Work out the finished part from the listing and answer in its coordinate system (mm). A direction names the side the tool comes from. Round coordinates to 2 decimals unless told otherwise and drop trailing zeros. Write each loop counter-clockwise with the first axis right and the second up, starting at its lowest first coordinate (ties: lowest second). Pieces come first, ordered by that corner, then holes. Notation, with made-up numbers: M 54.5,66.5 L 80.5,66.5 A32 cw 80.5,92.5 Z; hole C -39.75,18.5 d11. An arc over 180 degrees is marked long. One line per item, written item: value. Start each with the question number.
Q1. Find section A-A (y = -85). Write down the section's boundary in (x, z).
Q2. Find section B-B (x = -120.5). Write down the section's boundary in (y, z), and give its area (3 significant figures).
Q3. Find section D-D (z = -14). Write down the section's boundary in (x, y), and give its area (3 significant figures).
Q4. Consider probe 1 along X at (y, z) = (-78, 57.5); probe 2 along Z at (x, y) = (71.5, -64); probe 3 along Z at (x, y) = (-264, 102). Determine where each line is inside the solid, lowest interval first.
Q5. A tool of negligible diameter and unlimited length cuts with its end or side. For faces 4 (the flat face through (298, 8, 2)), 5 (the flat face through (4, 14, -225)), 6 (the flat face through (0, 115, -195)), 7 (the flat face through (-240, 55, -155)), 8 (the flat face through (299, -47, 3)), from which of +Z, -Z, +X, -X, +Y, -Y can it reach the whole face along a straight path? Write none if from no direction.
Q6. The mould has two halves that part along X. Classify faces 1 (the flat face through (-4, -47, 224)), 2 (the flat face through (-4, -36, 225)), 3 (the flat face through (300, -36, 3)): released by +X, released by -X, zero draft, split by the parting line, or undercut.
Q7. Find section C-C (y = 71). Write down the section's boundary in (x, z).
Q8. Given pin 1 Ø10 at (y, z) = (20.5, -154.5) entering from +X; pin 2 Ø10 at (x, z) = (-236.5, -150.5) entering from +Y; pin 3 Ø3 at (y, z) = (121.5, -202) entering from +X, each flat-ended and moving along its own axis, determine where each tip first touches the part or whether it passes through.
Autodesk Inventor part; units mm, degrees
ref_plane "YZ Plane" through (0, 0, 0) normal (1, 0, 0) x (0, 1, 0)
ref_plane "XZ Plane" through (0, 0, 0) normal (0, 1, 0) x (-1, 0, 0)
ref_plane "XY Plane" through (0, 0, 0) normal (0, 0, 1) x (1, 0, 0)
sketch "Sketch1" plane through (0, 0, 0) normal (0, 1, 0) x (-1, 0, 0)
  line L0 (-300, 225) -> (300, 225)
  line L1 (300, 225) -> (300, -225)
  line L2 (300, -225) -> (-300, -225)
  line L3 (-300, -225) -> (-300, 225)
  line L4 (-300, 225) -> (300, -225) construction
  line L5 (300, 225) -> (-300, -225) construction
  point P0 (0, 0)
  dimension "d0" = 600
  dimension "d1" = 450
extrude "Extrusion1" add sketch "Sketch1" along normal blind 5
sketch "Sketch6" plane through (0, 5, 0) normal (0, 1, 0) x (1, 0, 0)
  line L0 (300, 225) -> (-300, 225)
  line L1 (-300, -225) -> (300, -225)
  line L2 (300, -225) -> (300, 225)
  line L3 (300, 225) -> (-300, 225)
  line L4 (-300, 225) -> (-300, -225)
  line L5 (-300, -225) -> (300, 225) construction
  line L6 (300, -225) -> (-300, 225) construction
  line L7 (-298, -223.5) -> (298, -223.5)
  line L8 (298, -223.5) -> (298, 223.5)
  line L9 (298, 223.5) -> (-298, 223.5)
  line L10 (-298, 223.5) -> (-298, -223.5)
  line L11 (-298, -223.5) -> (298, 223.5) construction
  line L12 (298, -223.5) -> (-298, 223.5) construction
  point P0 (0, 0)
  dimension "d26" = 2
extrude "Extrusion7" add sketch "Sketch6" along normal blind 120
sketch "Sketch7" plane through (0, 0, 0) normal (0, -1, 0) x (1, 0, 0)
  line L0 (300, 225) -> (300, -225)
  line L1 (-300, 225) -> (300, 225)
  line L2 (300, 225) -> (300, -225)
  line L3 (300, -225) -> (-300, -225)
  line L4 (-300, -225) -> (-300, 225)
  line L5 (-300, 225) -> (300, -225) construction
  line L6 (300, 225) -> (-300, -225) construction
  point P0 (0, 0)
extrude "Extrusion8" add sketch "Sketch7" along normal blind 100
shell "Shell1" thickness 1 removed faces 1 at (-100, -100, 75)
mirror "Mirror1" about plane through (0, 0, 0) normal (0, 0, 1)
sketch "Sketch9" plane through (0, 125, 0) normal (0, 1, 0) x (1, 0, 0)
  line L0 (300, 225) -> (-300, 225)
  line L1 (-20, 225) -> (20, 225)
  line L2 (20, 225) -> (20, 175)
  line L3 (10, 165) -> (-10, 165)
  line L4 (-20, 175) -> (-20, 225)
  arc A0 (-20, 175) -> (-10, 165) centre (-10, 175) ccw
  arc A1 (10, 165) -> (20, 175) centre (10, 175) ccw
  point P0 (0, 0)
  point P1 (20, 165)
  point P2 (-20, 165)
  point P3 (0, 225)
  dimension "d37" = 40
  dimension "d38" = 60
  dimension "d39" = 10
extrude "Extrusion10" add sketch "Sketch9" against normal blind 10
sketch "Sketch10" plane through (0, 5, 0) normal (0, 1, 0) x (1, 0, 0)
  line L0 (-230, 165) -> (-250, 165)
  line L1 (-250, 165) -> (-250, 145)
  line L2 (-250, 145) -> (-230, 145)
  line L3 (-230, 145) -> (-230, 165)
  line L4 (-300, 225) -> (-300, -225)
  line L5 (300, 225) -> (-300, 225)
  point P0 (0, 0)
  point P1 (-250, 155)
  point P2 (-240, 165)
  dimension "d42" = 20
  dimension "d43" = 20
  dimension "d44" = 50
  dimension "d45" = 60
extrude "Extrusion11" add sketch "Sketch10" along normal blind 50
sketch "Sketch11" plane through (-298, 5, 223.5) normal (1, 0, 0) x (0, 0, -1)
  line L0 (448.5, 120) -> (448.5, -105)
  line L1 (0, 120) -> (448.5, 120)
  line L2 (448.5, 120) -> (448.5, 7.5)
  line L3 (448.5, 7.5) -> (0, 7.5)
  line L4 (0, 7.5) -> (0, 120)
  point P0 (223.5, -5)
extrude "Extrusion12" cut sketch "Sketch11" against normal through all
sketch "Sketch12" plane through (300, 125, 225) normal (1, 0, 0) x (0, 0, -1)
  line L0 (1.5, 0) -> (1.5, -112.5)
  line L1 (448.5, -120) -> (448.5, -112.5)
  line L2 (1.5, 0) -> (448.5, 0)
  line L3 (448.5, 0) -> (448.5, -112.5)
  line L4 (448.5, -112.5) -> (1.5, -112.5)
  line L5 (1.5, -112.5) -> (1.5, 0)
  point P0 (225, -125)
extrude "Extrusion13" cut sketch "Sketch12" against normal blind 10
sketch "Sketch13" plane through (-300, 125, 225) normal (0, 0, 1) x (1, 0, 0)
  line L0 (2, 0) -> (280, 0)
  line L1 (598, -120) -> (2, -120)
  line L2 (90, 0) -> (598, 0)
  line L3 (598, 0) -> (598, -120)
  line L4 (598, -120) -> (90, -120)
  line L5 (90, -120) -> (90, 0)
  line L6 (0, -225) -> (0, 0)
  point P0 (300, -125)
  point P1 (90, -120)
  dimension "d52" = 90
extrude "Extrusion14" cut sketch "Sketch13" against normal blind 10
sketch "Sketch14" plane through (298, 5, 225) normal (0, 0, 1) x (1, 0, 0)
  line L0 (-598, -105) -> (-598, 120)
  line L1 (-596, 0) -> (-508, 0)
  line L2 (-598, 120) -> (-578, 120)
  line L3 (-578, 120) -> (-578, 0)
  line L4 (-578, 0) -> (-598, 0)
  line L5 (-598, 0) -> (-598, 120)
  point P0 (-298, -5)
  dimension "d55" = 20
extrude "Extrusion15" cut sketch "Sketch14" against normal blind 10
sketch "Sketch15" plane through (300, -100, -225) normal (0, 0, -1) x (-1, 0, 0)
  point P0 (300, 100)
ref_plane "Work Plane1" through (0, 0, 0) normal (0, 0, 1) x (1, 0, 0)
properties part number "game base"
The answers:
1. outline: M -300,-225 L 300,-225 L 300,225 L -300,225 Z; hole M -299,-224 L 299,-224 L 299,224 L -299,224 Z
2. outline: M -100,-225 L 125,-225 L 125,-223.5 L 5,-223.5 L 5,225 L -100,225 L -100,224 L 4,224 L 4,-224 L -100,-224 Z
2. area: 838 mm2
3. outline: M -300,-100 L -299,-100 L -299,4 L 299,4 L 299,-100 L 300,-100 L 300,12.5 L 298,12.5 L 298,5 L -298,5 L -298,12.5 L -300,12.5 Z
3. area: 838 mm2
4. probe 1: -300 to -299, 299 to 300
4. probe 2: -225 to -224, 224 to 225
4. probe 3: -225 to -223.5, 223.5 to 225
5. face 4: +Z, +Y
5. face 5: -Z, +X, -X, +Y, -Y
5. face 6: +Z, +X, -X
5. face 7: +X, -X, +Y
5. face 8: -Y
6. face 1: undercut
6. face 2: zero draft
6. face 3: released by +X
7. outline: M -298,-225 L 300,-225 L 300,-223.5 L -298,-223.5 Z; M -280,223.5 L -210,223.5 L -210,225 L -280,225 Z; M 298,223.5 L 300,223.5 L 300,225 L 298,225 Z
8. pin 1: x = -230
8. pin 2: y = 55
8. pin 3: x = 20
